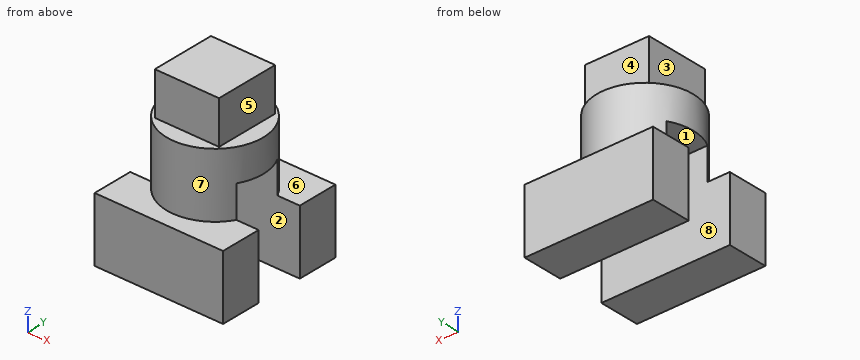
from build123d import *

# Parameters (mm, degrees)
F0_W     = 60
F0_H     = 60
F1_DEPTH = 30
F2_R     = 22.5
F3_DEPTH = 30
F4_W     = 30
F4_H     = 30
F5_DEPTH = 20
F6_W     = 22
F6_H     = 45
F7_DEPTH = 60


with BuildPart() as f1:
    # F0 (on Top) → F1 (new body)
    with BuildSketch(Plane.XY):
        Rectangle(F0_W, F0_H)
    extrude(amount=F1_DEPTH)

    # F2 (on face) → F3 (join)
    with BuildSketch(Plane.XY.offset(30)):
        Circle(F2_R)
    extrude(amount=F3_DEPTH)

    # F4 (on face) → F5 (join)
    with BuildSketch(Plane.XY.offset(60)):
        Rectangle(F4_W, F4_H)
    extrude(amount=F5_DEPTH)

    # F6 (on face) → F7 (cut)
    with BuildSketch(Plane.YZ.offset(30)):
        with Locations((0, 22.5)):
            Rectangle(F6_W, F6_H)
    extrude(amount=-F7_DEPTH, mode=Mode.SUBTRACT)


solid = f1.part
Design review of the part built by this model. Coordinates are the model's own, in mm. Face numbers are marked on the shaded views. A direction names the side the tool comes from. Coordinates: 2 decimals unless noted, no trailing zeros. Write each loop counter-clockwise with the first axis right and the second up, starting at its lowest first coordinate (ties: lowest second). Pieces come first, ordered by that corner, then holes. Notation, with made-up numbers: (80, 55) - (138, 55) arc R23 cw to (138, 89) - close; hole circle Ø4 at (46, 42). An arc over 180 degrees is marked (long way). One line per item, written item: value.
1) Mouldability with a two-part tool opening along Y and no side actions: class the marked faces 1, 2, 3 and 4 as +Y half, -Y half, draft (parallel to the pull), parting line (faces both ways), or undercut.
Answer sheet:
face 1: undercut
face 2: undercut
face 3: draft
face 4: +Y half
2) Add section C-C (y = 0). State the section outline as (x, z) points.
Answer sheet:
outline: (-22.5, 45) - (22.5, 45) - (22.5, 60) - (15, 60) - (15, 80) - (-15, 80) - (-15, 60) - (-22.5, 60) - close
3) Add section A-A (x = -26). State the section outline as (y, z) points.
Answer sheet:
outline: (-30, 0) - (-11, 0) - (-11, 30) - (-30, 30) - close; (11, 0) - (30, 0) - (30, 30) - (11, 30) - close
4) Add section B-B (z = 24). State the section outline as (x, y) points, plus the area to 3 significant figures.
Answer sheet:
outline: (-30, -30) - (30, -30) - (30, -11) - (-30, -11) - close; (-30, 11) - (30, 11) - (30, 30) - (-30, 30) - close
area: 2,280 mm2
5) For the marked faces 5, 6, 7 and 8, list the 3-axis set-ups (+Z, -Z, +X, -X, +Y, -Y) from which the entire face can be reached by the end or side of a thin tool; tool diameter is ignored.
Answer sheet:
face 5: +Z, +X, +Y, -Y
face 6: +Z, +Y
face 7: +Z
face 8: -Z, +X, -X
6) To check wall thickness, follow probe 1 along Y at (x, z) = (-17.5, 27.5); probe 2 along Z at (x, y) = (17, 22); probe 3 along Z at (x, y) = (-2, 20.5). State the ranges of each line that lie inside material, in increasing order.
Answer sheet:
probe 1: y = -30 to -11, 11 to 30
probe 2: z = 0 to 30
probe 3: z = 0 to 60
7) Add section D-D (x = -1). State the section outline as (y, z) points.
Answer sheet:
outline: (-30, 0) - (-11, 0) - (-11, 45) - (11, 45) - (11, 0) - (30, 0) - (30, 30) - (22.48, 30) - (22.48, 60) - (15, 60) - (15, 80) - (-15, 80) - (-15, 60) - (-22.48, 60) - (-22.48, 30) - (-30, 30) - close
8) Insertion check: pin 1 (17.5 mm diameter, centred on x = 4, y = -0.5, fed in from -Z); pin 2 (12 mm diameter, centred on x = 17.5, y = 18, fed in from -Z); pin 3 (10 mm diameter, centred on y = 7.5, z = 70, fed in from +X); pin 4 (1.5 mm diameter, centred on x = -8.5, z = 31.5, fed in from -Y). Each pin has a flat end and moves straight along its axis. Give the tip position at first contact, or say it passes through.
Answer sheet:
pin 1: stops at z = 45
pin 2: stops at z = 0
pin 3: stops at x = 15
pin 4: stops at y = -21.12
